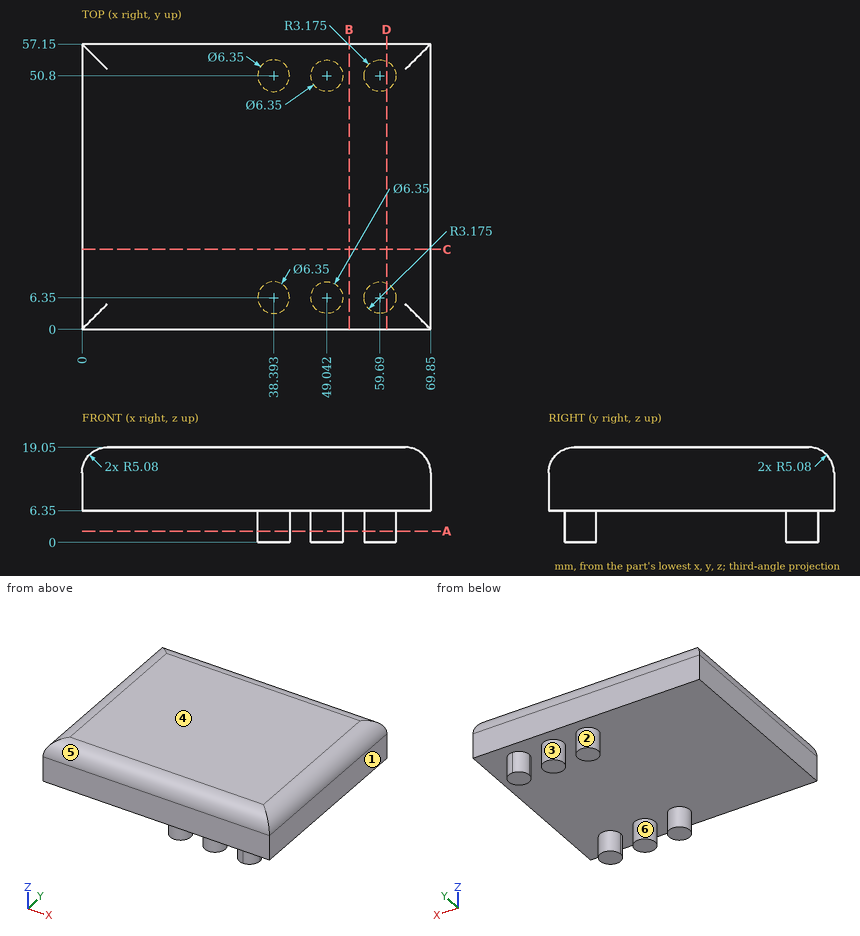
Drawing for the job (mm, zero at the part's lowest x, y, z). A direction names the side the tool comes from. Give positions to 0.01 mm unless a question says otherwise; leave off trailing zeros. Write each loop counter-clockwise with the first axis right and the second up, starting at its lowest first coordinate (ties: lowest second). Pieces come first, ordered by that corner, then holes. Notation, with made-up numbers: M -6.75,-8 L 3.25,-8 A12 ccw 3.25,10 Z; hole C 62.25,16.5 d10. An arc over 180 degrees is marked long. Return JSON: item names as keys, results as strings. Group by question number.
(1) Drill centre lines: L1, parallel to Z at x = 21.5, y = 13; L2, parallel to Y at x = 57, z = 2.25 (1 decimal); L3, parallel to Y at x = 37, z = 17.75 (1 decimal). Where is each one in solid material? Low to high. Write a range as [from, to].
(2) Band-saw the part on A-A (z = 2.25). State how many separate pieces and enclosed holes the cut face has, and give its area (3 significant figures).
(3) 3-axis set-ups, long thin cutter, end or side, ignore diameter. For the marked faces 5 and 6: which of +Z, -Z, +X, -X, +Y, -Y reach the whole face in a straight line?
(4) Band-saw the part on C-C (y = 16). Give the cut face in (x, z).
(5) Band-saw the part on B-B (x = 53.5). Give the cut face in (y, z), and give its area (3 significant figures).
(6) Mould opens along X. For the marked faces 1, 2, 3 and 4 say: pulls with the +X half, pulls with the -X half, needs draft (parallel to the pull), parting line crosses it, or undercut.
(7) Flat gauge pin, fed straight in: pin 1 Ø10 at (x, y) = (61, 42.5) entering from -Z. Where does the tip first touch, or does it go through?
(8) Band-saw the part on D-D (x = 61). Give the cut face in (y, z).
Entries:
{
 "1": {"L1": "z = [6.35, 19.05]", "L2": "y = [4.7, 8], [49.1, 52.5]", "L3": "y = [1.7, 55.5]"},
 "2": {"separate pieces": "6", "enclosed holes": "0", "area": "190 mm^2"},
 "3": {"face 5": "+Z, +X, -X, -Y", "face 6": "-Z"},
 "4": {"outline": "M 0,6.35 L 69.85,6.35 L 69.85,13.97 A5.08 ccw 64.77,19.05 L 5.08,19.05 A5.08 ccw 0,13.97 Z"},
 "5": {"outline": "M 0,6.35 L 57.15,6.35 L 57.15,13.97 A5.08 ccw 52.07,19.05 L 5.08,19.05 A5.08 ccw 0,13.97 Z", "area": "715 mm^2"},
 "6": {"face 1": "pulls with the +X half", "face 2": "undercut", "face 3": "undercut", "face 4": "needs draft"},
 "7": {"pin 1": "stops at z = 6.35"},
 "8": {"outline": "M 0,6.35 L 3.46,6.35 L 3.46,0 L 9.24,0 L 9.24,6.35 L 47.91,6.35 L 47.91,0 L 53.69,0 L 53.69,6.35 L 57.15,6.35 L 57.15,13.97 A5.08 ccw 52.07,19.05 L 5.08,19.05 A5.08 ccw 0,13.97 Z"}
}
